```python
from build123d import *

# Parameters (mm, degrees)
CYLINDER004_R     = 3
CYLINDER004_DEPTH = 10
PAD010_DEPTH      = 10
SKETCH036_R       = 1.75
POCKET025_DEPTH   = 45.001
CHAMFER023_1_SIZE = 3
CHAMFER023_2_SIZE = 2
CHAMFER023_3_SIZE = 1
CHAMFER024_SIZE   = 0.5


with BuildPart() as boardbracketscrewheadcylinder001:
    # Cylinder004 → Cylinder004 (new body)
    with BuildSketch(Plane(origin=(0, 0.5, 24), x_dir=(1, 0, 0), z_dir=(0, 0, 1))):
        Circle(CYLINDER004_R)
    extrude(amount=CYLINDER004_DEPTH)


with BuildPart() as obj1:
    # Sketch035 → Pad010 (new body, symmetric)
    with BuildSketch(Plane.YZ):
        Polygon((4.5, 21), (4.5, 24), (-0.12132, 28.62132), (-5.071068, 33.571068), (-7.545942, 31.096194), (-6.838835, 30.389087), (-5.778175, 31.449747), (-4.717514, 30.389087), (-6.131728, 28.974874), (-2.949747, 25.792893), (-35.476659, -6.734019), (-38.65864, -3.552038), (-40.072853, -4.966252), (-41.133514, -3.905592), (-40.072853, -2.844931), (-40.77996, -2.137825), (-43.254834, -4.612698), (-38.305087, -9.562446), (-36.183766, -11.683766), (-25.12132, -0.62132), (-4.742641, -21), (4.5, -21), (4.5, -18), (-3.5, -18), (-23, 1.5), (-3.5, 21), align=None)
    extrude(amount=PAD010_DEPTH, both=True)

    # Cut002: cut BoardBracketScrewHeadCylinder001
    add(boardbracketscrewheadcylinder001.part, mode=Mode.SUBTRACT)

    # Sketch036 → Pocket025 (cut, through all)
    with BuildSketch(Plane.XY.offset(24)):
        with Locations((0, 0.5)):
            Circle(SKETCH036_R)
    extrude(amount=-POCKET025_DEPTH, mode=Mode.SUBTRACT)

    # Chamfer023 1
    chamfer023_1_edges = [obj1.edges().sort_by_distance(p)[0] for p in [
        (0, -36.183766, -11.683766),
    ]]
    chamfer(chamfer023_1_edges, length=CHAMFER023_1_SIZE)

    # Chamfer023 2
    chamfer023_2_edges = [obj1.edges().sort_by_distance(p)[0] for p in [
        (0, -25.12132, -0.62132),
    ]]
    chamfer(chamfer023_2_edges, length=CHAMFER023_2_SIZE)

    # Chamfer023 3
    chamfer023_3_edges = [obj1.edges().sort_by_distance(p)[0] for p in [
        (0, -35.476659, -6.734019),
        (0, -43.254834, -4.612698),
        (0, -5.071068, 33.571068),
    ]]
    chamfer(chamfer023_3_edges, length=CHAMFER023_3_SIZE)

    # Chamfer024
    chamfer024_edges = [obj1.edges().sort_by_distance(p)[0] for p in [
        (10, -5.424621, 29.681981),
        (10, -39.365747, -4.259145),
        (10, -5.247845, 30.919417),
        (10, -40.603184, -4.435922),
        (10, 4.5, 22.5),
        (10, 0.5, 21),
        (10, -13.25, 11.25),
        (10, -13.25, -8.25),
        (10, 0.5, -18),
        (10, 4.5, -19.5),
    ]]
    chamfer(chamfer024_edges, length=CHAMFER024_SIZE)


solid = obj1.part
```
The listing builds one solid part. Answer for the finished solid, in the listing's coordinates (mm). A direction names the side the tool comes from. Coordinates: 2 decimals unless noted, no trailing zeros. Loops run counter-clockwise (first coordinate to the right, second up) from the corner with the lowest first, then second, coordinate; pieces in that order, holes last. Notation, with made-up numbers: (55, -20) -> (87, -20) arc R21 ccw to (87, -10) -> close; hole circle Ø1 at (16, 73.25). An arc over 180 degrees is marked (long way). Return JSON: item names as keys, results as strings. Group by question number.
(1) A cutting plane is placed at B-B on x = 0. Count the separate pieces of the cut face and the enclosed holes in it, and give its area (3 significant figures).
(2) A cutting plane is placed at C-C on y = -17. Write down the section's boundary in (x, z), and give its area (3 significant figures).
(3) Which of the six approach directions +Z, -Z, +X, -X, +Y, -Y give full straight-line access (tool end or side, diameter ignored) to faces 1 (the flat face through (-0.1, -13.4, 11.1)), 2 (the flat face through (0, -35, -6.027)), 3 (the flat face through (0.14, -14.358, -11.385))?
(4) Determine the mould class of faces 4 (the cylindrical face through (-0.65, -2.43, 26.7)), 5 (the flat face through (9.75, -40.75, -4.64)), 6 (the flat face through (0, 4.5, -20)) for opening direction X: released by +X, released by -X, zero draft, split by the parting line, or undercut.
(5) A cutting plane is placed at A-A on y = 0.5. Write down the section's boundary in (x, z).
(6) Given pin 1 Ø5 at (x, z) = (-1.5, 20) entering from -Y; pin 2 Ø4.5 at (x, y) = (0, 0.5) entering from -Z; pin 3 Ø3 at (x, y) = (4, -35) entering from +Z; pin 4 Ø4 at (x, z) = (0.5, -14) entering from +Y, each flat-ended and moving along its own axis, determine where each tip first touches the part or whether it passes through.
(7) Find the intervals of material crossed by probe 1 along Z at (x, y) = (-1.75, 2); probe 2 along Z at (x, y) = (-5.25, -6); probe 3 along X at (y, z) = (0.5, 25.5), in increasing order. Write a range as from..to.
The answers:
{
 "1": {"separate pieces": "3", "enclosed holes": "0", "area": "299 mm^2"},
 "2": {"outline": "(-10, -8.74) -> (10, -8.74) -> (10, -5.21) -> (9.5, -4.5) -> (-10, -4.5) -> close; (-10, 7.5) -> (9.5, 7.5) -> (10, 8.21) -> (10, 11.74) -> (-10, 11.74) -> close", "area": "169 mm^2"},
 "3": {"face 1": "+X, -X, +Y", "face 2": "+Z, +X, -X", "face 3": "-Z, +X, -X"},
 "4": {"face 4": "undercut", "face 5": "released by +X", "face 6": "zero draft"},
 "5": {"outline": "(-10, -21) -> (-1.75, -21) -> (-1.75, -18) -> (-10, -18) -> close; (-10, 21) -> (-1.75, 21) -> (-1.75, 24) -> (-3, 24) -> (-3, 28) -> (-10, 28) -> close; (1.75, -21) -> (10, -21) -> (10, -18.5) -> (9.5, -18) -> (1.75, -18) -> close; (1.75, 21) -> (9.5, 21) -> (10, 21.5) -> (10, 28) -> (3, 28) -> (3, 24) -> (1.75, 24) -> close"},
 "6": {"pin 1": "stops at y = -11.24", "pin 2": "stops at z = -21", "pin 3": "stops at z = -4.76", "pin 4": "stops at y = -5.5"},
 "7": {"probe 1": "z = -21..-18, 21..24", "probe 2": "z = -19.74..-15.5, 18.5..22.74, 28.84..29.11, 31.23..32.64", "probe 3": "x = -10..-3, 3..10"}
}
